```python
from build123d import *

# Parameters (mm, degrees)
SKETCH1_W                   = 127
SKETCH1_H                   = 19.05
BOSS_EXTRUDE1_DEPTH         = 50.8
F_1_2_CLEARANCE_HOLE1_D     = 13.49248
F_3_8_16_TAPPED_HOLE1_D     = 7.9375
F_12_24_TAPPED_HOLE1_D      = 4.4958
F_1_4_0_25_DIAMETER_HOLE1_D = 6.35


with BuildPart() as part:
    # Sketch1 → Boss-Extrude1 (new body)
    with BuildSketch(Plane.XY):
        with Locations((63.5, 9.525)):
            Rectangle(SKETCH1_W, SKETCH1_H)
    extrude(amount=BOSS_EXTRUDE1_DEPTH)

    # 1/2 Clearance Hole1 (through all)
    with Locations(Plane(origin=(0, 19.05, 0), x_dir=(1, 0, 0), z_dir=(0, 1, 0))):
        with Locations((25.4, -25.4)):
            Hole(F_1_2_CLEARANCE_HOLE1_D / 2)

    # 3/8-16 Tapped Hole1 (through all)
    with Locations(Plane(origin=(0, 19.05, 0), x_dir=(1, 0, 0), z_dir=(0, 1, 0))):
        with Locations((50.8, -25.4)):
            Hole(F_3_8_16_TAPPED_HOLE1_D / 2)

    # #12-24 Tapped Hole1 (through all)
    with Locations(Plane(origin=(0, 19.05, 0), x_dir=(1, 0, 0), z_dir=(0, 1, 0))):
        with Locations((76.2, -25.4)):
            Hole(F_12_24_TAPPED_HOLE1_D / 2)

    # 1/4 (0.25) Diameter Hole1 (through all)
    with Locations(Plane(origin=(0, 19.05, 0), x_dir=(1, 0, 0), z_dir=(0, 1, 0))):
        with Locations((101.6, -25.4)):
            Hole(F_1_4_0_25_DIAMETER_HOLE1_D / 2)


solid = part.part
```
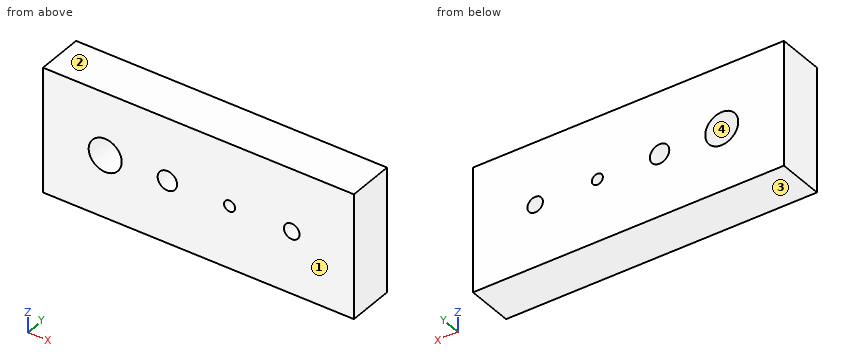
Geometry: final body of the model. Coordinates: model frame, mm. Face numbers are marked on the shaded views. Give positions to 0.01 mm unless a question says otherwise; leave off trailing zeros. Loops run counter-clockwise (first coordinate to the right, second up) from the corner with the lowest first, then second, coordinate; pieces in that order, holes last. Notation, with made-up numbers: (23, 37) -> (65, 37) arc R6 cw to (65, 46) -> close; hole circle Ø3 at (33.25, 38.25). An arc over 180 degrees is marked (long way). Return JSON: item names as keys, results as strings.
Item 1: Section C-C, the plane z = 25.4. Output: boundary loops of the cut face in (x, y) (3 decimals).
Filled in:
{"outline": "(0, 0) -> (18.654, 0) -> (18.654, 19.05) -> (0, 19.05) -> close; (32.146, 0) -> (46.831, 0) -> (46.831, 19.05) -> (32.146, 19.05) -> close; (54.769, 0) -> (73.952, 0) -> (73.952, 19.05) -> (54.769, 19.05) -> close; (78.448, 0) -> (98.425, 0) -> (98.425, 19.05) -> (78.448, 19.05) -> close; (104.775, 0) -> (127, 0) -> (127, 19.05) -> (104.775, 19.05) -> close"}
Item 2: Mould query, pull axis Z, two halves, no side actions, for the marked faces 1, 2, 3 and 4. Classes: released by +Z, released by -Z, zero draft, split by the parting line, or undercut.
Filled in:
{"face 1": "zero draft", "face 2": "released by +Z", "face 3": "released by -Z", "face 4": "undercut"}
Item 3: Line query: line 1 (X direction, y = 9.75, z = 25.4) (3 decimals); line 2 (Z direction, x = 25.4, y = 9); line 3 (Z direction, x = 76, y = 7). Output: solid intervals per line, ascending.
Filled in:
{"line 1": "0 to 18.654, 32.146 to 46.831, 54.769 to 73.952, 78.448 to 98.425, 104.775 to 127", "line 2": "0 to 18.65, 32.15 to 50.8", "line 3": "0 to 23.16, 27.64 to 50.8"}
Item 4: Section A-A, the plane x = 76.2. Output: boundary loops of the cut face in (y, z), plus the area to 3 significant figures.
Filled in:
{"outline": "(0, 0) -> (19.05, 0) -> (19.05, 23.15) -> (0, 23.15) -> close; (0, 27.65) -> (19.05, 27.65) -> (19.05, 50.8) -> (0, 50.8) -> close", "area": "882 mm^2"}
Item 5: Section B-B, the plane y = 14. Count the separate pieces of the cut face and the enclosed holes in it, plus the area to 3 significant figures.
Filled in:
{"separate pieces": "1", "enclosed holes": "4", "area": "6,210 mm^2"}
Item 6: Section D-D, the plane x = 25.4. Output: boundary loops of the cut face in (y, z).
Filled in:
{"outline": "(0, 0) -> (19.05, 0) -> (19.05, 18.65) -> (0, 18.65) -> close; (0, 32.15) -> (19.05, 32.15) -> (19.05, 50.8) -> (0, 50.8) -> close"}
Item 7: Pin query (flat end, axial travel): P1, Ø2.5, axis at x = 76.2, z = 25.4, coming from the +Y side. Return the tip coordinate at first contact, or that it passes through.
Filled in:
{"P1": "through"}
